For this review, take the finished solid that the model builds, in its own axes (mm). Give positions to 0.01 mm unless a question says otherwise; leave off trailing zeros. Order: outer loops, then holes, each group sorted by start corner. A loop starts at its lowest first (then second) coordinate and runs counter-clockwise, first axis right, second up. Notation, with made-up numbers: (40.5, 7) -> (54.5, 7) arc R26 ccw to (54.5, 39) -> close; hole circle Ø5 at (-23.75, 78). An arc over 180 degrees is marked (long way). Return JSON: item names as keys, results as strings. Group by question number.
1) Add section A-A (y = 7). Give the boundary of the cut face in (x, z).
2) Add section C-C (z = -0.15). Give the boundary of the cut face in (x, y), then the cut area to 3 significant figures.
3) To check wall thickness, follow line 1 along Y through (x, z) = (-3, -0.5); line 2 along Y through (x, z) = (-2.75, -0.25); line 3 along X through (y, z) = (-10, 0.3). State the ranges of each line that lie inside material, in increasing order.
4) The part is to be moulded in two halves that separate along X. For faces 1 (the face through (-2.56, -8.92, -0.01)), 2 (the face through (-2.71, -11.85, 0.01)), 3 (the face through (2.71, -11.85, 0.01)), 4 (the face through (-1.5, -8.3, -0.6)), say which applies: released by +X, released by -X, zero draft, split by the parting line, or undercut.
5) Add section D-D (y = -5.25). Give the boundary of the cut face in (x, z), then the cut area to 3 significant figures.
6) Add section B-B (x = 2). Give the boundary of the cut face in (y, z).
7) Insertion check: P1, Ø1.8, axis at x = -2.43, y = -9.91, coming from the -Z side; P2, Ø2.5, axis at x = 2.43, y = -9.91, coming from the -Z side. Each pin has a flat end and moves straight along its axis. Give the tip position at first contact, or say it passes through.
from build123d import *

# Parameters (mm, degrees)
SKETCH4_R           = 1
BOSS_EXTRUDE1_DEPTH = 0.6
FILLET1_R           = 2.065056386
FILLET2_R           = 0.516264097


with BuildPart() as part:
    # Sketch4 → Boss-Extrude1 (new, symmetric)
    with BuildSketch(Plane.XY):
        with BuildLine():
            Line((-5.246180053, -10.967229122), (-5.356700553, -7.785130647))
            ThreePointArc((-5.356700553, -7.785130647), (-9.598805691, 3.443313149), (0, 10.65))
            Line((0, 10.65), (0, 8.25))
            ThreePointArc((0, 8.25), (-8.248743485, 0.143982353), (-0.287920848, -8.244974323))
            Line((-0.287920848, -8.244974323), (-0.424287349, -12.15))
            ThreePointArc((-0.424287349, -12.15), (-2.896253939, -11.807380441), (-5.246180053, -10.967229122))
        make_face()
        with Locations((-2.430824062, -9.909926787)):
            Circle(SKETCH4_R, mode=Mode.SUBTRACT)
    extrude(amount=BOSS_EXTRUDE1_DEPTH, both=True)

    # Fillet1
    fillet1_edges = [part.edges().sort_by_distance(p)[0] for p in [
        (-5.356700553, -7.785130647, 0),
    ]]
    fillet(fillet1_edges, radius=FILLET1_R)

    # Fillet2
    fillet2_edges = [part.edges().sort_by_distance(p)[0] for p in [
        (-5.246180053, -10.967229122, 0),
    ]]
    fillet(fillet2_edges, radius=FILLET2_R)

    # Mirror1: part across plane


with BuildPart() as part_1:
    add(part.part)
    add(part.part.mirror(Plane(origin=(0, 10.65, 0.6), x_dir=(0, 0, 1), z_dir=(-1, 0, 0))))


solid = part_1.part
Evaluation:
{
 "1": {"outline": "(-7.72, -0.6) -> (-4.37, -0.6) -> (-4.37, 0.6) -> (-7.72, 0.6) -> close; (4.37, -0.6) -> (7.72, -0.6) -> (7.72, 0.6) -> (4.37, 0.6) -> close"},
 "2": {"outline": "(-6.12, -7.25) arc R2.07 cw to (-5.32, -8.81) -> (-5.26, -10.65) arc R0.52 ccw to (-4.95, -11.1) arc R12.16 ccw to (-0.42, -12.15) -> (-0.29, -8.24) arc R8.25 cw (long way) to (0.29, -8.24) -> (0.42, -12.15) arc R12.16 ccw to (4.95, -11.1) arc R0.52 ccw to (5.26, -10.65) -> (5.32, -8.81) arc R2.07 cw to (6.12, -7.25) arc R10 ccw (long way) to start; hole circle Ø2 at (-2.43, -9.91); hole circle Ø2 at (2.43, -9.91)", "area": "122 mm^2"},
 "3": {"line 1": "-11.78 to -10.73, -9.09 to -7.69, 7.69 to 10.19", "line 2": "-11.84 to -10.86, -8.96 to -7.78, 7.78 to 10.26", "line 3": "-5.28 to -3.43, -1.43 to -0.35, 0.35 to 1.43, 3.43 to 5.28"},
 "4": {"face 1": "undercut", "face 2": "released by -X", "face 3": "released by +X", "face 4": "zero draft"},
 "5": {"outline": "(-8.07, -0.6) -> (-6.36, -0.6) -> (-6.36, 0.6) -> (-8.07, 0.6) -> close; (6.36, -0.6) -> (8.07, -0.6) -> (8.07, 0.6) -> (6.36, 0.6) -> close", "area": "4.08 mm^2"},
 "6": {"outline": "(-11.99, -0.6) -> (-10.81, -0.6) -> (-10.81, 0.6) -> (-11.99, 0.6) -> close; (-9.01, -0.6) -> (-8, -0.6) -> (-8, 0.6) -> (-9.01, 0.6) -> close; (8, -0.6) -> (10.45, -0.6) -> (10.45, 0.6) -> (8, 0.6) -> close"},
 "7": {"P1": "through", "P2": "z = -0.6"}
}
